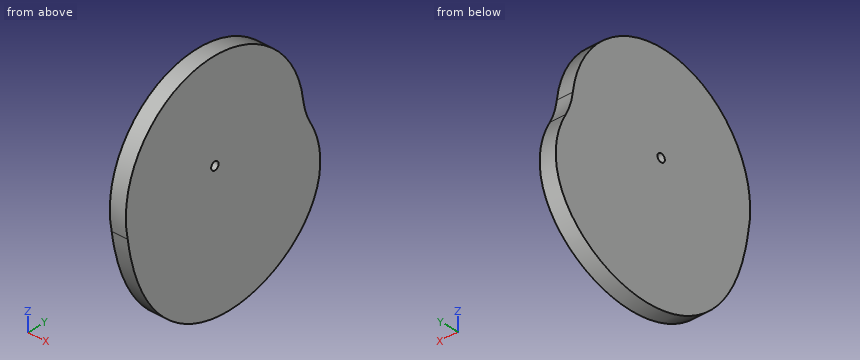
Autodesk Inventor part; units mm, degrees
ref_plane "YZ Plane" through (0, 0, 0) normal (1, 0, 0) x (0, 1, 0)
ref_plane "XZ Plane" through (0, 0, 0) normal (0, 1, 0) x (-1, 0, 0)
ref_plane "XY Plane" through (0, 0, 0) normal (0, 0, 1) x (1, 0, 0)
sketch "Sketch1" plane through (0, 0, 0) normal (1, 0, 0) x (0, 1, 0)
  circle A0 centre (0, 0) radius 76.2
  spline S0 degree 3 poles (76.2, 0) (145.5168, -95.878) (-64.2426, -180.0292) (-76.2, 0) knots 0 0 0 0 1 1 1 1
  point P0 (76.2, -76.2)
  point P1 (0, -105.0953)
  dimension "d0" = 152.4
extrude "Extrusion1" add sketch "Sketch1" along normal blind 12.7
fillet "Fillet1" radius 50.8 1 edges at (6.35, 76.2, 0)
sketch "Sketch2" plane through (12.7, 0, 0) normal (1, 0, 0) x (0, 0, -1)
  arc A0 (-9.8256, 75.5639) -> (0, -76.2) centre (0, 0) ccw
hole "Hole1" at (12.7, 0, 0) direction (-1, 0, 0) diameter 6.35 end through all
properties part number "plateCamPart"
Build history of the part. All positions in model axes, mm. Round coordinates to 2 decimals unless told otherwise and drop trailing zeros. Order: outer loops, then holes, each group sorted by start corner. A loop starts at its lowest first (then second) coordinate and runs counter-clockwise, first axis right, second up. Notation, with made-up numbers: (8, -35) - (22, -35) arc R14 ccw to (22, -19) - close; hole circle Ø8 at (8.5, -32). An arc over 180 degrees is marked (long way). Use a Markdown table: item, result.
1) Flat gauge pins, fed straight in: pin 1 Ø5 at (x, y) = (6.5, 7) entering from +Z; pin 2 Ø6 at (y, z) = (1, -41.5) entering from -X; pin 3 Ø4 at (x, z) = (2, -86.5) entering from +Y; pin 4 Ø2 at (x, z) = (7, -82.5) entering from -Y. Where does each tip first touch, or does it go through?
Recorded:
| item | result |
|---|---|
| pin 1 | stops at z = 76.07 |
| pin 2 | stops at x = 0 |
| pin 3 | stops at y = 68.08 |
| pin 4 | stops at y = -46.27 |
2) Saw through at A-A on z = 40. Write the cut outline in (x, y), and give its area (3 significant figures).
Recorded:
| item | result |
|---|---|
| outline | (0, -64.86) - (12.7, -64.86) - (12.7, 64.86) - (0, 64.86) - close |
| area | 1,650 mm² |
3) Wall check: L1, parallel to Y at x = 5.25, z = 0 (3 decimals); L2, parallel to Z at x = 10.25, y = 0 (3 decimals); L3, parallel to Y at x = 10.25, z = -6.5. Give the ranges that are in metal, low to high.
Recorded:
| item | result |
|---|---|
| L1 | y = -76.2 to -3.175, 3.175 to 77.852 |
| L2 | z = -105.095 to -3.175, 3.175 to 76.2 |
| L3 | y = -75.92 to 80.58 |
